Input: part model. Units: mm. Frame: model coordinates. Give positions to 0.01 mm unless a question says otherwise; leave off trailing zeros. Loops run counter-clockwise (first coordinate to the right, second up) from the corner with the lowest first, then second, coordinate; pieces in that order, holes last.
from build123d import *

# Parameters (mm, degrees)
F0_W     = 19
F0_H     = 14
F1_DEPTH = 3
F2_W     = 0.75
F2_H     = 0.75
F3_DEPTH = 1.5
F5_DEPTH = 14.001
F7_DEPTH = 5.127709538
F8_R     = 0.59999


# Not quite as in the source:
# - a fillet or chamfer is up to 0.001 mm smaller than in the source, because OpenCascade refuses the exact size


with BuildPart() as f1:
    # F0 (on Top) → F1 (new body)
    with BuildSketch(Plane.XY):
        Rectangle(F0_W, F0_H)
    extrude(amount=F1_DEPTH)

    # F2 (on face) → F3 (join)
    with BuildSketch(Plane(origin=(0, 0, 0), x_dir=(1, 0, 0), z_dir=(0, 0, -1))):
        with Locations((9.125, 6.625)):
            Rectangle(F2_W, F2_H)
        with Locations((-9.125, 6.625)):
            Rectangle(F2_W, F2_H)
        with Locations((-9.125, -6.625)):
            Rectangle(F2_W, F2_H)
        with Locations((9.125, -6.625)):
            Rectangle(F2_W, F2_H)
    extrude(amount=F3_DEPTH)

    # F4 (on face) → F5 (cut, through all)
    with BuildSketch(Plane.XZ.offset(7)):
        Polygon((-3.773290462, 3), (-4.973290462, 3), (-4.373290462, 2.4), align=None)
    extrude(amount=-F5_DEPTH, mode=Mode.SUBTRACT)

    # F6 (on face) → F7 (cut, through all)
    with BuildSketch(Plane(origin=(-9.5, 0, 0), x_dir=(0, -1, 0), z_dir=(-1, 0, 0))):
        Polygon((0.6, 3), (-0.6, 3), (0, 2.4), align=None)
    extrude(amount=-F7_DEPTH, mode=Mode.SUBTRACT)

    # F8 (radius 0.6 in the source; OpenCascade refuses exactly that, so slightly less here)
    f8_edges = [f1.edges().sort_by_distance(p)[0] for p in [
        (-3.77329, 0, 3),
        (-4.97329, 3.8, 3),
        (-4.97329, -3.8, 3),
        (-7.236645, -0.6, 3),
        (-7.236645, 0.6, 3),
        (2.863355, -7, 3),
        (-7.236645, -7, 3),
        (2.863355, 7, 3),
        (9.5, 0, 3),
        (-7.236645, 7, 3),
        (-9.5, 3.8, 3),
        (-9.5, -3.8, 3),
    ]]
    fillet(f8_edges, radius=F8_R)


solid = f1.part
(1) Cut plane A-A (z = -0.85). Return the cut outline in (x, y), and give its area (3 significant figures).
Values follow:
outline: (-9.5, -7) - (-8.75, -7) - (-8.75, -6.25) - (-9.5, -6.25) - close; (-9.5, 6.25) - (-8.75, 6.25) - (-8.75, 7) - (-9.5, 7) - close; (8.75, -7) - (9.5, -7) - (9.5, -6.25) - (8.75, -6.25) - close; (8.75, 6.25) - (9.5, 6.25) - (9.5, 7) - (8.75, 7) - close
area: 2.25 mm2
(2) Pin query (flat end, axial travel): pin 1 Ø4 at (x, y) = (0, -3.5) entering from -Z. Return the tip coordinate at first contact, or that it passes through.
Values follow:
pin 1: stops at z = 0
(3) Cut plane C-C (x = -6). Return the cut outline in (y, z), and give its area (3 significant figures).
Values follow:
outline: (-7, 0) - (7, 0) - (7, 2.4) arc R0.6 ccw to (6.4, 3) - (0.85, 3) arc R0.6 ccw to (0.42, 2.82) - (0, 2.4) - (-0.42, 2.82) arc R0.6 ccw to (-0.85, 3) - (-6.4, 3) arc R0.6 ccw to (-7, 2.4) - close
area: 41.5 mm2
(4) Cut plane B-B (y = 1.25). Return the cut outline in (x, z), and give its area (3 significant figures).
Values follow:
outline: (-9.5, 0) - (9.5, 0) - (9.5, 2.4) arc R0.6 ccw to (8.9, 3) - (-3.52, 3) arc R0.6 ccw to (-3.95, 2.82) - (-4.37, 2.4) - (-4.8, 2.82) arc R0.6 ccw to (-5.22, 3) - (-8.9, 3) arc R0.6 ccw to (-9.5, 2.4) - close
area: 56.5 mm2
(5) Ray query, probe 1 along Z at (x, y) = (1, -5); probe 2 along X at (y, z) = (-6, 2.7); probe 3 along X at (y, z) = (-4.5, 2.6). Return the intervals inside material, ascending.
Values follow:
probe 1: z = 0 to 3
probe 2: x = -9.42 to -4.67, -4.07 to 9.42
probe 3: x = -9.47 to -4.57, -4.17 to 9.47
(6) Cut plane D-D (x = 3.25). Return the cut outline in (y, z), and give its area (3 significant figures).
Values follow:
outline: (-7, 0) - (7, 0) - (7, 2.4) arc R0.6 ccw to (6.4, 3) - (-6.4, 3) arc R0.6 ccw to (-7, 2.4) - close
area: 41.8 mm2
